Could you check a few things on this model? Use its own coordinates, in mm. A direction names the side the tool comes from. Give positions to 0.01 mm unless a question says otherwise; leave off trailing zeros. Write each loop counter-clockwise with the first axis right and the second up, starting at its lowest first coordinate (ties: lowest second). Pieces come first, ordered by that corner, then holes. Notation, with made-up numbers: M 39.25,51.25 L 57.25,51.25 A29 ccw 57.25,75.25 Z; hole C 8.25,46.25 d7. An arc over 180 degrees is marked long. One line per item, written item: value.
```python
from build123d import *

# Parameters (mm, degrees)
CHANFRO2_SIZE = 0.2


with BuildPart() as part:
    # Esboço1 → Revolução1 (revolve)
    with BuildSketch(Plane.XY, mode=Mode.PRIVATE) as revolu_o1_sk:
        Polygon((13, 0), (59, 0), (59, 7.1), (56, 7.1), (56, 5.5), (52.5, 5.5), (52.5, 7.1), (40.5, 7.1), (36, 3.3), (0, 3.3), (0, 1.85), (13, 1.85), align=None)
    revolve(revolu_o1_sk.sketch.rotate(Axis((13, 0, 0), (1, 0, 0)), 90), axis=Axis((13, 0, 0), (1, 0, 0)))

    # Chanfro2
    chanfro2_edges = [part.edges().sort_by_distance(p)[0] for p in [
        (0, 0, -3.3),
        (52.5, 0, -7.1),
        (56, 0, -7.1),
        (59, 0, -7.1),
    ]]
    chamfer(chanfro2_edges, length=CHANFRO2_SIZE)


solid = part.part
```
1) We'd pull the mould along Y, two halves only. Please class faces 1 (the face through (13, 0, 0)), 2 (the face through (46.32, -7.04, -0.92)), 3 (the face through (56, 3, -5)): pulls with the +Y half, pulls with the -Y half, needs draft (parallel to the pull), parting line crosses it, or undercut.
Outcome:
face 1: undercut
face 2: parting line crosses it
face 3: needs draft
2) I'm going to push flat-ended pins straight in: pin 1 (8 mm diameter, centred on x = 34.5, y = 4, fed in from -Z); pin 2 (1.5 mm diameter, centred on x = 48, z = -2.5, fed in from +Y); pin 3 (3 mm diameter, centred on y = -1, z = -4, fed in from -X); pin 4 (1 mm diameter, centred on y = 3.5, z = 3, fed in from -X). Where does each tip first touch, or does it pass through?
Outcome:
pin 1: stops at z = -4.55
pin 2: stops at y = 6.88
pin 3: stops at x = 0
pin 4: stops at x = 36.96
3) On a 3-axis mill with a long thin cutter (end or side, diameter ignored), from which of +Z, -Z, +X, -X, +Y, -Y can I reach the whole of each face in a straight line? I mean faces 4 (the face through (0, 2.02, -0.04)), 5 (the face through (6.591, 1.806, -0.401)), 6 (the face through (52.5, 3, 5)). Say none if no direction works.
Outcome:
face 4: +Z, -Z, -X, +Y, -Y
face 5: -X
face 6: none
4) Please list where these lines run through material, in increasing order: L1, parallel to Y at x = 8.5, z = 0; L2, parallel to X at y = -4.5, z = -4; L3, parallel to X at y = -2.5, z = 6.25. Write a range as from..to.
Outcome:
L1: y = -3.3..-1.85, 1.85..3.3
L2: x = 39.22..52.5, 56..59
L3: x = 40.06..52.5, 56..59
5) If we section it at A-A, the plane y = 0: Write out the boundary of the cut face in (x, z), then the cut area to 3 significant figures.
Outcome:
outline: M 0,-3.1 L 0.2,-3.3 L 36,-3.3 L 40.5,-7.1 L 52.3,-7.1 L 52.5,-6.9 L 52.5,-5.5 L 56,-5.5 L 56,-6.9 L 56.2,-7.1 L 58.8,-7.1 L 59,-6.9 L 59,6.9 L 58.8,7.1 L 56.2,7.1 L 56,6.9 L 56,5.5 L 52.5,5.5 L 52.5,6.9 L 52.3,7.1 L 40.5,7.1 L 36,3.3 L 0.2,3.3 L 0,3.1 L 0,1.85 L 13,1.85 L 13,-1.85 L 0,-1.85 Z
area: 488 mm^2
6) If we section it at C-C, the plane x = 55.5: Write out the boundary of the cut face in (y, z), then the cut area to 3 significant figures.
Outcome:
outline: C 0,0 d11
area: 95.0 mm^2
7) If we section it at D-D, the plane x = 4: Write out the boundary of the cut face in (y, z).
Outcome:
outline: C 0,0 d6.6; hole C 0,0 d3.7
